Input: part model. Units: mm. Frame: model coordinates. A direction names the side the tool comes from. Give positions to 0.01 mm unless a question says otherwise; leave off trailing zeros. Loops run counter-clockwise (first coordinate to the right, second up) from the corner with the lowest first, then second, coordinate; pieces in that order, holes last. Notation, with made-up numbers: M -31.5,42.5 L 15.5,42.5 A8 cw 15.5,54.5 Z; hole C 37,-35 d2. An arc over 180 degrees is marked long. One line per item, written item: value. Start each with the question number.
(1) Ray query, line 1 along X through (y, z) = (-98.5, -1.5); line 2 along X through (y, z) = (-99.5, 12); line 3 along X through (y, z) = (-9, 9). Return the intervals inside material, ascending. Write a range as from..to.
(2) Section C-C on y = -27. Output: boundary loops of the cut face in (x, z), plus the area to 3 significant figures.
(3) Pull-direction query (X, two-part tool) for faces 4 (the flat face through (0, -160, 0)), 5 (the flat face through (19, -86, 3.794)), 6 (the flat face through (-30, -71, 0)); classes: released by +X, released by -X, zero draft, split by the parting line, or undercut.
(4) Section A-A on z = 12.5. Output: boundary loops of the cut face in (x, y), plus the area to 3 significant figures.
(5) Section B-B on y = 0. Output: boundary loops of the cut face in (x, z).
(6) Section D-D on z = -2. Output: boundary loops of the cut face in (x, y).
(7) Access query for faces 1 (the flat face through (24.654, 0.28, -7.605)), 2 (the flat face through (11.372, -91.26, -5.735)), 3 (the flat face through (0, 5, -12)). Directions: +Z, -Z, +X, -X, +Y, -Y. A direction counts if a zero-diameter tool reaches every point of the face in a straight line with its end or side. Return the directions, or none.
(8) Pin query (flat end, axial travel): P1, Ø4, axis at x = -17, z = 8.5, coming from the -Y side. Return the tip coordinate at first contact, or that it passes through.
```python
from build123d import *

# Parameters (mm, degrees)
F1_DEPTH = 160
F2_W     = 10
F2_H     = 10
F3_DEPTH = 60
F5_DEPTH = 60


with BuildPart() as f1:
    # F0 (on Front) → F1 (new body, symmetric)
    with BuildSketch(Plane.XZ):
        Polygon((30, -15), (30, 15), (-8, 15), (-14.8404028665, -3.7938524157), (-22.8404028665, -3.7938524157), (-16, 15), (-30, 15), (-30, -15), (8, -15), (14.8404028665, 3.7938524157), (22.8404028665, 3.7938524157), (16, -15), align=None)
    extrude(amount=F1_DEPTH, both=True)

    # F2 (on face) → F3 (cut)
    with BuildSketch(Plane.XY.offset(15)):
        Rectangle(F2_W, F2_H)
    extrude(amount=-F3_DEPTH, mode=Mode.SUBTRACT)

    # F4 (on face) → F5 (intersect)
    with BuildSketch(Plane.YZ.offset(30)):
        Polygon((0, 7.5), (0, 15), (-160, 15), (-160, -15), (0, -15), (0, -7.5), (-20, 0), align=None)
        Polygon((20, 15), (0, 15), (0, 7.5), align=None)
        Polygon((0, -15), (20, -15), (0, -7.5), align=None)
    extrude(amount=-F5_DEPTH, mode=Mode.INTERSECT)


solid = f1.part
```
Output values:
1. line 1: x = -30..-22.01, -14.01..12.91, 20.91..30
1. line 2: x = -30..-17.09, -9.09..30
1. line 3: x = -30..-18.18, -10.18..30
2. outline: M -30,-15 L 8,-15 L 14.84,3.79 L 22.84,3.79 L 16,-15 L 30,-15 L 30,15 L -8,15 L -14.84,-3.79 L -22.84,-3.79 L -16,15 L -30,15 Z
2. area: 1,500 mm²
3. face 4: zero draft
3. face 5: undercut
3. face 6: released by -X
4. outline: M -30,-160 L -16.91,-160 L -16.91,13.33 L -30,13.33 Z; M -8.91,-160 L 30,-160 L 30,13.33 L -8.91,13.33 Z; hole M -5,-5 L 5,-5 L 5,5 L -5,5 Z
4. area: 8,910 mm²
5. outline: M -30,-15 L -5,-15 L -5,-7.5 L -30,-7.5 Z; M -30,7.5 L -18.73,7.5 L -16,15 L -30,15 Z; M -10.73,7.5 L -5,7.5 L -5,15 L -8,15 Z; M 5,-15 L 8,-15 L 10.73,-7.5 L 5,-7.5 Z; M 5,7.5 L 30,7.5 L 30,15 L 5,15 Z; M 16,-15 L 30,-15 L 30,-7.5 L 18.73,-7.5 Z
6. outline: M -30,-160 L -22.19,-160 L -22.19,-14.67 L -30,-14.67 Z; M -14.19,-160 L 12.73,-160 L 12.73,-14.67 L -14.19,-14.67 Z; M 20.73,-160 L 30,-160 L 30,-14.67 L 20.73,-14.67 Z
7. face 1: +X, -X, +Y
7. face 2: -Z, +Y, -Y
7. face 3: +Z, -Z
8. P1: stops at y = -160
